from build123d import *

# Parameters (mm, degrees)
SKETCH1_W           = 97.58
SKETCH1_H           = 200.21
BOSS_EXTRUDE1_DEPTH = 43.58
SKETCH2_W           = 2
SKETCH2_H           = 148.11
CUT_EXTRUDE1_DEPTH  = 1
SKETCH3_W           = 148.11
SKETCH3_H           = 1
CUT_EXTRUDE2_DEPTH  = 100
SKETCH4_W           = 93.58
SKETCH4_H           = 50.6
CUT_EXTRUDE4_DEPTH  = 40.58
SKETCH5_W           = 93.58
SKETCH5_H           = 148.11
CUT_EXTRUDE5_DEPTH  = 39.58
SKETCH6_R           = 12
CUT_EXTRUDE6_DEPTH  = 39.58
SKETCH7_R           = 30.26
CUT_EXTRUDE7_DEPTH  = 39.58
SKETCH10_W          = 148.11
SKETCH10_H          = 3
BOSS_EXTRUDE2_DEPTH = 13.15
SKETCH11_W          = 148.11
SKETCH11_H          = 3
BOSS_EXTRUDE3_DEPTH = 13.15


with BuildPart() as part:
    # Sketch1 → Boss-Extrude1 (new body)
    with BuildSketch(Plane(origin=(0, 0, 0), x_dir=(1, 0, 0), z_dir=(0, 1, 0))):
        with Locations((48.79, 100.105)):
            Rectangle(SKETCH1_W, SKETCH1_H)
    extrude(amount=BOSS_EXTRUDE1_DEPTH)

    # Sketch2 → Cut-Extrude1 (cut)
    with BuildSketch(Plane.XZ):
        with Locations((1, -126.155)):
            Rectangle(SKETCH2_W, SKETCH2_H)
    extrude(amount=-CUT_EXTRUDE1_DEPTH, mode=Mode.SUBTRACT)

    # Sketch3 → Cut-Extrude2 (cut)
    with BuildSketch(Plane.ZY.offset(-2)):
        with Locations((-126.155, 0.5)):
            Rectangle(SKETCH3_W, SKETCH3_H)
    extrude(amount=-CUT_EXTRUDE2_DEPTH, mode=Mode.SUBTRACT)

    # Sketch4 → Cut-Extrude4 (cut)
    with BuildSketch(Plane(origin=(0, 0, 0), x_dir=(-1, 0, 0), z_dir=(0, -1, 0))):
        with Locations((-48.79, 26.8)):
            Rectangle(SKETCH4_W, SKETCH4_H)
    extrude(amount=-CUT_EXTRUDE4_DEPTH, mode=Mode.SUBTRACT)

    # Sketch5 → Cut-Extrude5 (cut)
    with BuildSketch(Plane(origin=(0, 1, 0), x_dir=(-1, 0, 0), z_dir=(0, -1, 0))):
        with Locations((-48.79, 126.155)):
            Rectangle(SKETCH5_W, SKETCH5_H)
    extrude(amount=-CUT_EXTRUDE5_DEPTH, mode=Mode.SUBTRACT)

    # Sketch6 → Cut-Extrude6 (cut)
    with BuildSketch(Plane.XY):
        with Locations((50.746792762, 5.57)):
            Circle(SKETCH6_R)
    extrude(amount=-CUT_EXTRUDE6_DEPTH, mode=Mode.SUBTRACT)

    # Sketch7 → Cut-Extrude7 (cut)
    with BuildSketch(Plane(origin=(0, 43.58, 0), x_dir=(1, 0, 0), z_dir=(0, 1, 0))):
        with Locations(Location((49.98, 34.51, 0), (0, 0, 270))):
            Circle(SKETCH7_R)
    extrude(amount=-CUT_EXTRUDE7_DEPTH, mode=Mode.SUBTRACT)

    # Sketch10 → Boss-Extrude2 (add)
    with BuildSketch(Plane.ZY):
        with Locations((-126.155, 2.5)):
            Rectangle(SKETCH10_W, SKETCH10_H)
    extrude(amount=BOSS_EXTRUDE2_DEPTH)

    # Sketch11 → Boss-Extrude3 (add)
    with BuildSketch(Plane(origin=(97.58, 0, 0), x_dir=(0, 0, -1), z_dir=(1, 0, 0))):
        with Locations((126.155, 2.5)):
            Rectangle(SKETCH11_W, SKETCH11_H)
    extrude(amount=BOSS_EXTRUDE3_DEPTH)


solid = part.part
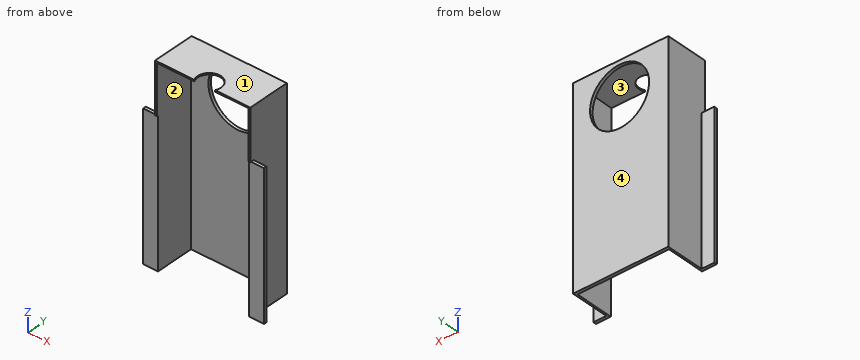
For this review, take the finished solid that the model builds, in its own axes (mm). Face numbers are marked on the shaded views. A direction names the side the tool comes from. Round coordinates to 2 decimals unless told otherwise and drop trailing zeros. Write each loop counter-clockwise with the first axis right and the second up, starting at its lowest first coordinate (ties: lowest second). Pieces come first, ordered by that corner, then holes. Notation, with made-up numbers: (52, 22) - (75, 22) arc R11 ccw to (75, 34) - close; hole circle Ø1 at (-22, 6.5). An arc over 180 degrees is marked (long way). Use a Markdown table: item, result.
Q1. Clearance check with flat-ended pins moving along their axes: pin 1 (12 mm diameter, centred on y = 24.5, z = -110, fed in from -X); pin 2 (1.5 mm diameter, centred on x = 91, z = -30, fed in from -Y); pin 3 (0.5 mm diameter, centred on x = 96.5, y = 0.5, fed in from -Z); pin 4 (19 mm diameter, centred on x = 50.75, y = 5.57, fed in from -Z). State where each tip first meets the part, or that it passes through.
Derived:
| item | result |
|---|---|
| pin 1 | stops at x = 0 |
| pin 2 | stops at y = 40.58 |
| pin 3 | stops at z = -52.1 |
| pin 4 | passes through |
Q2. Machinability: for the marked faces 3 and 4, which of the approach directions +Z, -Z, +X, -X, +Y, -Y give a long, thin tool a straight path to every point of the face, cutting with its end or side? Answer none if there is none.
Derived:
| item | result |
|---|---|
| face 3 | -Z, -Y |
| face 4 | +Z, -Z, +X, -X, +Y |
Q3. Wall thickness on line 1 along X through (y, z) = (42.7, -34.51); line 2 along X through (y, z) = (31.5, -56); line 3 along Y through (x, z) = (87.5, -90): over which ranges is each line inside the solid? List them lowest first.
Derived:
| item | result |
|---|---|
| line 1 | x = 0 to 19.72, 80.24 to 97.58 |
| line 2 | x = 0 to 2, 95.58 to 97.58 |
| line 3 | y = 40.58 to 43.58 |
Q4. We need section C-C (z = -91). Give the boundary of the cut face in (x, y).
Derived:
| item | result |
|---|---|
| outline | (-13.15, 1) - (2, 1) - (2, 40.58) - (95.58, 40.58) - (95.58, 1) - (110.73, 1) - (110.73, 4) - (97.58, 4) - (97.58, 43.58) - (0, 43.58) - (0, 4) - (-13.15, 4) - close |
Q5. We need section D-D (x = 49.98). Give the boundary of the cut face in (y, z), plus the area to 3 significant figures.
Derived:
| item | result |
|---|---|
| outline | (17.55, -1.5) - (40.58, -1.5) - (40.58, -4.25) - (43.58, -4.25) - (43.58, 0) - (17.55, 0) - close; (40.58, -200.21) - (43.58, -200.21) - (43.58, -64.77) - (40.58, -64.77) - close |
| area | 454 mm2 |
Q6. We need section A-A (z = -34.51). Give the boundary of the cut face in (x, y), plus the area to 4 significant figures.
Derived:
| item | result |
|---|---|
| outline | (0, 0) - (2, 0) - (2, 40.58) - (19.72, 40.58) - (19.72, 43.58) - (0, 43.58) - close; (80.24, 40.58) - (95.58, 40.58) - (95.58, 0) - (97.58, 0) - (97.58, 43.58) - (80.24, 43.58) - close |
| area | 273.5 mm2 |
Q7. We need section B-B (y = 38). Give the boundary of the cut face in (x, z), plus the area to 3 significant figures.
Derived:
| item | result |
|---|---|
| outline | (0, -200.21) - (2, -200.21) - (2, -1.5) - (95.58, -1.5) - (95.58, -200.21) - (97.58, -200.21) - (97.58, 0) - (0, 0) - close |
| area | 941 mm2 |
Q8. The part is to be moulded in two halves that separate along X. For the marked faces 1 and 2, say which applies: pulls with the +X half, pulls with the -X half, needs draft (parallel to the pull), parting line crosses it, or undercut.
Derived:
| item | result |
|---|---|
| face 1 | needs draft |
| face 2 | undercut |
